Verification items for the finished model (mm, model axes). A direction names the side the tool comes from. Give positions to 0.01 mm unless a question says otherwise; leave off trailing zeros. Loops run counter-clockwise (first coordinate to the right, second up) from the corner with the lowest first, then second, coordinate; pieces in that order, holes last. Notation, with made-up numbers: M 51,81.5 L 58,81.5 A26 ccw 58,117.5 Z; hole C 66.25,64 d6. An arc over 180 degrees is marked long. Use a Markdown table: item, result.
from build123d import *

# Parameters (mm, degrees)
BOSS_EXTRUDE1_DEPTH = 10


with BuildPart() as part:
    # Sketch1 → Boss-Extrude1 (new body)
    with BuildSketch(Plane.XY):
        with BuildLine():
            Line((9.875388203, 0), (-9.875388203, 0))
            ThreePointArc((-9.875388203, 0), (-17.450099602, 10.83745824), (-30, 15))
            ThreePointArc((-30, 15), (-31.8749625, 15.255779094), (-33.612903226, 16.004424108))
            ThreePointArc((-33.612903226, 16.004424108), (-33.896535204, 16.29613728), (-34, 16.689632781))
            Line((-34, 16.689632781), (-34, 17.162645351))
            ThreePointArc((-34, 17.162645351), (-33.578745661, 17.867309614), (-32.75862069, 17.829866682))
            ThreePointArc((-32.75862069, 17.829866682), (-25.031925557, 22.564124391), (-33.623370468, 25.445458816))
            ThreePointArc((-33.623370468, 25.445458816), (-33.953767859, 25.215558804), (-34.348044562, 25.134550579))
            Line((-34.348044562, 25.134550579), (-34.791587602, 25.134550579))
            ThreePointArc((-34.791587602, 25.134550579), (-35.51482586, 25.592605522), (-35.409856969, 26.442234524))
            ThreePointArc((-35.409856969, 26.442234524), (-29.220414383, 28.95645357), (-23.74103901, 25.134550579))
            Line((-23.74103901, 25.134550579), (-5, 5.145359938))
            Line((-5, 5.145359938), (5, 5.145359938))
            Line((5, 5.145359938), (23.74103901, 25.134550579))
            ThreePointArc((23.74103901, 25.134550579), (29.220414383, 28.95645357), (35.409856969, 26.442234524))
            ThreePointArc((35.409856969, 26.442234524), (35.51482586, 25.592605522), (34.791587602, 25.134550579))
            Line((34.791587602, 25.134550579), (34.348044562, 25.134550579))
            ThreePointArc((34.348044562, 25.134550579), (33.953767859, 25.215558804), (33.623370468, 25.445458816))
            ThreePointArc((33.623370468, 25.445458816), (25.031925557, 22.564124391), (32.75862069, 17.829866682))
            ThreePointArc((32.75862069, 17.829866682), (33.578745661, 17.867309614), (34, 17.162645351))
            Line((34, 17.162645351), (34, 16.689632781))
            ThreePointArc((34, 16.689632781), (33.896535204, 16.29613728), (33.612903226, 16.004424108))
            ThreePointArc((33.612903226, 16.004424108), (31.8749625, 15.255779094), (30, 15))
            ThreePointArc((30, 15), (17.450099602, 10.83745824), (9.875388203, 0))
        make_face()
    extrude(amount=BOSS_EXTRUDE1_DEPTH)


solid = part.part
(1) Cross-section at D-D on x = 17.5. Record the cut outline in (y, z).
Results below:
| item | result |
|---|---|
| outline | M 10.87,0 L 18.48,0 L 18.48,10 L 10.87,10 Z |
(2) Material ranges on line 1 (Y direction, x = 30, z = 2.25); line 2 (Y direction, x = 1, z = 1.5); line 3 (X direction, y = 22, z = 5.25), recorded low to high.
Results below:
| item | result |
|---|---|
| line 1 | 15 to 17, 27 to 29 |
| line 2 | 0 to 5.15 |
| line 3 | -25 to -20.8, 20.8 to 25 |
(3) Gauge pin test, flat ends, axial feed: P1, Ø3, axis at x = -20, z = 7.5, coming from the -Y side; P2, Ø3, axis at x = -2, z = 5, coming from the +Y side; P3, Ø6, axis at x = 21, z = 1, coming from the -Y side. Record the tip position at first contact, or that the pin passes through.
Results below:
| item | result |
|---|---|
| P1 | y = 11.57 |
| P2 | y = 5.15 |
| P3 | y = 11.23 |
(4) Cross-section at B-B on x = 27. Record the cut outline in (y, z).
Results below:
| item | result |
|---|---|
| outline | M 14.78,0 L 18,0 L 18,10 L 14.78,10 Z; M 26,0 L 28.32,0 L 28.32,10 L 26,10 Z |
(5) Cross-section at C-C on z = 8. Record the cut outline in (x, y), then the cut area to 3 significant figures.
Results below:
| item | result |
|---|---|
| outline | M -35.41,26.44 A0.8 ccw -34.79,25.13 L -34.35,25.13 A1 ccw -33.62,25.45 A5 cw long -32.76,17.83 A0.8 ccw -34,17.16 L -34,16.69 A0.8 ccw -33.61,16 A7 ccw -30,15 A21 cw -9.88,0 L 9.88,0 A21 cw 30,15 A7 ccw 33.61,16 A0.8 ccw 34,16.69 L 34,17.16 A0.8 ccw 32.76,17.83 A5 cw long 33.62,25.45 A1 ccw 34.35,25.13 L 34.79,25.13 A0.8 ccw 35.41,26.44 A7 ccw 23.74,25.13 L 5,5.15 L -5,5.15 L -23.74,25.13 A7 ccw Z |
| area | 485 mm^2 |
(6) Set-up check for faces 1 (the cylindrical face through (-17.3, 10.724, 4.93)), 2 (the flat face through (14.24, 15, 4.93)), 3 (the cylindrical face through (33.57, 17.87, 4.93)): record each of +Z, -Z, +X, -X, +Y, -Y from which the full face is reachable in a straight line by a thin tool's end or side.
Results below:
| item | result |
|---|---|
| face 1 | +Z, -Z, -X, -Y |
| face 2 | +Z, -Z, +Y |
| face 3 | +Z, -Z |
(7) Cross-section at A-A on y = 13. Record the cut outline in (x, z).
Results below:
| item | result |
|---|---|
| outline | M -21.06,0 L -12.36,0 L -12.36,10 L -21.06,10 Z; M 12.36,0 L 21.06,0 L 21.06,10 L 12.36,10 Z |
(8) Draft check along Y on faces 4 (the cylindrical face through (25.052, 22.722, 4.93)), 5 (the cylindrical face through (-29.317, 28.967, 4.93)), 6 (the cylindrical face through (-33.59, 17.86, 4.93)), 7 (the cylindrical face through (31.901, 15.263, 4.93)). Enter one of: +Y half, -Y half, draft (parallel to the pull), parting line (faces both ways), or undercut.
Results below:
| item | result |
|---|---|
| face 4 | undercut |
| face 5 | +Y half |
| face 6 | undercut |
| face 7 | -Y half |
